Read the model definition and answer for the solid it produces. Units are mm, in the model's axes. A direction names the side the tool comes from. Coordinates: 2 decimals unless noted, no trailing zeros. Order: outer loops, then holes, each group sorted by start corner. A loop starts at its lowest first (then second) coordinate and runs counter-clockwise, first axis right, second up. Notation, with made-up numbers: (-29.75, 10.5) - (-19.75, 10.5) arc R28 ccw to (-19.75, 43.5) - close; hole circle Ø10 at (73.5, 51). An arc over 180 degrees is marked (long way). Use one line per item in the form item = value. Start each with the question number.
Autodesk Inventor part; units mm, degrees
ref_plane "YZ Plane" through (0, 0, 0) normal (1, 0, 0) x (0, 1, 0)
ref_plane "XZ Plane" through (0, 0, 0) normal (0, 1, 0) x (-1, 0, 0)
ref_plane "XY Plane" through (0, 0, 0) normal (0, 0, 1) x (1, 0, 0)
sketch "Base" plane through (0, 0, 0) normal (0, 1, 0) x (-1, 0, 0)
  line L0 (0, 35) -> (0, -175)
  line L1 (0, -175) -> (65, -175)
  line L2 (65, -175) -> (65, 35)
  line L3 (65, 35) -> (0, 35)
  dimension "d6" = 210
  dimension "d7" = 65
extrude "Extrusion2" add sketch "Base" along normal blind 65
sketch "Top" plane through (0, 65, 0) normal (0, 1, 0) x (1, 0, 0)
  circle A0 centre (-32.5, 46) radius 17
  circle A1 centre (-32.5, -2) radius 17
  circle A2 centre (-32.5, 94) radius 17
  circle A3 centre (-32.5, 142) radius 17
  line L0 (0, 175) -> (-65, 175)
  line L1 (-65, 175) -> (-65, -35)
  line L2 (-65, -35) -> (0, -35) construction
  line L3 (-32.5, -35) -> (-32.5, 175) construction
  circle A4 centre (-32.5, -2) radius 15
  circle A5 centre (-32.5, 46) radius 15
  circle A6 centre (-32.5, 94) radius 15
  circle A7 centre (-32.5, 142) radius 15
  point P0 (-32.5, 70)
  dimension "d10" = 34
  dimension "d11" = 34
  dimension "d12" = 34
  dimension "d13" = 34
  dimension "d14" = 48
  dimension "d15" = 48
  dimension "d16" = 48
  dimension "d27" = 30
  dimension "d28" = 30
  dimension "d29" = 30
  dimension "d30" = 30
  dimension "d31" = 24
  dimension "d32" = 105
  dimension "d35" = 33
extrude "Extrusion3" cut sketch "Top" against normal up to next contours A4 | A5 | A6 | A7
sketch "Walls" plane through (0, 0, 0) normal (0, -1, 0) x (1, 0, 0)
  line L0 (-11, 24) -> (-54, 24)
  line L1 (-54, 24) -> (-54, -164)
  line L2 (-54, -164) -> (-11, -164)
  line L3 (-11, -164) -> (-11, 24)
  line L4 (-65, 35) -> (0, 35)
  line L5 (0, -175) -> (-65, -175)
  line L6 (0, 35) -> (0, -175)
  line L7 (-65, -175) -> (-65, 35)
  point P0 (0, 0)
  dimension "d21" = 11
  dimension "d22" = 11
  dimension "d23" = 11
  dimension "d24" = 11
  dimension "d33" = 43
  dimension "d47" = 65
extrude "Extrusion4" cut sketch "Walls" against normal blind 48.5 contours L3 L2 L1 L0
sketch "Sketch6" plane through (0, 0, 35) normal (1, 0, 0) x (0, 0, -1)
  line L0 (0, 0) -> (210, 0)
  line L1 (11, 48.5) -> (199, 48.5)
  point P0 (35, 0)
  point P1 (33.3852, 33.5)
  dimension "d34" = 48.5
fillet "Fillet1" radius 6 8 edges at (-32.5, 65, 35) (-65, 65, -70) (0, 65, -70) (0, 32.5, 35) (-65, 32.5, 35) (0, 32.5, -175) (-32.5, 65, -175) (-65, 32.5, -175)
sketch "Sketch7" plane through (-65, 0, -169) normal (-1, 0, 0) x (0, 0, 1)
  line L0 (0, 59) -> (198, 59)
  line L1 (99, 59) -> (99, 0) construction
  line L2 (0, 0) -> (198, 0)
  circle A0 centre (99, 0) radius 6.35
  point P0 (169, 0)
  dimension "d40" = 12.7
extrude "Extrusion5" cut sketch "Sketch7" against normal up to surface (11 mm away)
fillet "Fillet2" radius 6 4 edges at (-11, 24.25, 24) (-54, 24.25, 24) (-11, 24.25, -164) (-54, 24.25, -164)
sketch "Sketch8" plane through (0, 0, 29) normal (1, 0, 0) x (0, 0, -1)
  line L0 (0, 0) -> (198, 0)
  line L1 (198, 65) -> (0, 65)
  point P0 (29, 0)
  dimension "d42" = 65
fillet "Fillet3" radius 1.5 8 edges at (-52.2426, 48.5, 22.2426) (-32.5, 48.5, 24) (-12.7574, 48.5, 22.2426) (-11, 48.5, -70) (-12.7574, 48.5, -162.2426) (-32.5, 48.5, -164) (-52.2426, 48.5, -162.2426) (-54, 48.5, -70)
sketch "Sketch9" plane through (0, 0, 0) normal (0, -1, 0) x (1, 0, 0)
  line L0 (-54, -63.65) -> (-54, 18)
  line L1 (-11, 18) -> (-11, -158)
  line L2 (-65, -63.65) -> (-54, -63.65)
  line L3 (-54, -76.35) -> (-65, -76.35)
  line L4 (-48, 24) -> (-17, 24)
  point P0 (0, 0)
  dimension "d44" = 43
  dimension "d45" = 12.7
  dimension "d46" = 87.65
sketch "Sketch11" plane through (-6, 0, -175) normal (0, 0, -1) x (-1, 0, 0)
  line L0 (84.0226, 97.8745) -> (-43.2429, 97.8745)
  line L1 (-43.2429, 97.8745) -> (-43.2429, -59.4459)
  line L2 (-43.2429, -59.4459) -> (84.0226, -59.4459)
  line L3 (84.0226, -59.4459) -> (84.0226, 97.8745)
  point P0 (-6, 0)
extrude "Extrusion7" cut sketch "Sketch11" against normal blind 105
equation "\"d8\" = d7"
equation "\"d11\" = d10"
equation "\"d12\" = d10"
equation "\"d13\" = d10"
equation "\"d15\" = d14"
equation "\"d16\" = d14"
equation "\"d28\" = d27"
equation "\"d29\" = d27"
equation "\"d30\" = d27"
equation "\"d22\" = d21"
equation "\"d23\" = d21"
equation "\"d24\" = d23"
equation "\"d25\" = d7 - 1.5 * d21"
equation "\"d41\" = d36"
equation "\"d43\" = 0.25 * d36"
equation "\"d50\" = 0.5 * d6"
properties part number "Full"
Q1. For a pull along X with two mould halves and no side action, classify faces 4 (the cylindrical face through (-63.196, 63.289, -19.807)), 5 (the flat face through (-25, 55, -70)), 6 (the cylindrical face through (-43.556, 56.866, -56.138)) as +X half, -X half, draft (parallel to the pull), parting line (faces both ways), or undercut.
Q2. A cutting plane is placed at C-C (z = -46). Give the vertices of the cut face in (x, y), then the cut area to 3 significant figures.
Q3. A cutting plane is placed at A-A (x = -32.5). Give the vertices of the cut face in (y, z), then the cut area to 3 significant figures.
Q4. Given P1, Ø6, axis at x = -44.5, y = 19, coming from the -Z side; P2, Ø1, axis at x = -43.5, z = -22, coming from the -Y side; P3, Ø5, axis at x = -45, y = 45, coming from the -Z side, each flat-ended and moving along its own axis, determine where each tip first touches the part or whether it passes through.
Q5. Consider probe 1 along Z at (x, y) = (-32.5, 56.75); probe 2 along X at (y, z) = (41, -16); probe 3 along X at (y, z) = (59, -46). Determine where each line is inside the solid, lowest interval first.
Q6. A cutting plane is placed at B-B (y = 54.5). Give the vertices of the cut face in (x, z).
Q7. A cutting plane is placed at D-D (y = 34). Give the vertices of the cut face in (x, z).
Q8. Which of the six approach directions +Z, -Z, +X, -X, +Y, -Y give full straight-line access (tool end or side, diameter ignored) to faces 1 (the cylindrical face through (-12.804, 23.829, 22.289)), 2 (the flat face through (-32, 65, -20)), 3 (the cylindrical face through (-59.58, 4.44, -65.46))?
Result sheet:
q1.face_4 = -X half
q1.face_5 = draft
q1.face_6 = undercut
q2.outline = (-65, 0) - (-54, 0) - (-54, 47) arc R1.5 cw to (-52.5, 48.5) - (-47.5, 48.5) - (-47.5, 65) - (-59, 65) arc R6 ccw to (-65, 59) - close; (-17.5, 48.5) - (-12.5, 48.5) arc R1.5 cw to (-11, 47) - (-11, 0) - (0, 0) - (0, 59) arc R6 ccw to (-6, 65) - (-17.5, 65) - close
q2.area = 1,630 mm^2
q3.outline = (0, 24) - (47, 24) arc R1.5 cw to (48.5, 22.5) - (48.5, 17) - (65, 17) - (65, 29) arc R6 ccw to (59, 35) - (0, 35) - close; (48.5, -70) - (65, -70) - (65, -61) - (48.5, -61) - close; (48.5, -31) - (65, -31) - (65, -13) - (48.5, -13) - close
q3.area = 1,270 mm^2
q4.P1 = 24
q4.P2 = 48.5
q4.P3 = 23.91
q5.probe_1 = -70 to -61, -31 to -13, 17 to 35
q5.probe_2 = -65 to -54, -11 to 0
q5.probe_3 = -65 to -47.5, -17.5 to 0
q6.outline = (-65, -70) - (0, -70) - (0, 29) arc R6 ccw to (-6, 35) - (-59, 35) arc R6 ccw to (-65, 29) - close; hole circle Ø30 at (-32.5, -46); hole circle Ø30 at (-32.5, 2)
q7.outline = (-65, -70) - (-54, -70) - (-54, 18) arc R6 cw to (-48, 24) - (-17, 24) arc R6 cw to (-11, 18) - (-11, -70) - (0, -70) - (0, 29) arc R6 ccw to (-6, 35) - (-59, 35) arc R6 ccw to (-65, 29) - close
q8.face_1 = -Z, -Y
q8.face_2 = +Z, -Z, +X, -X, +Y
q8.face_3 = -Z, -X, -Y
